from build123d import *

# Parameters (mm, degrees)
SKETCH1_W           = 2.9718
SKETCH1_H           = 12.7
SKETCH1_W_2         = 63.5
SKETCH1_H_2         = 31.75
SKETCH1_W_3         = 25.4
SKETCH1_H_3         = 2.739734253
BOSS_EXTRUDE1_DEPTH = 2.9718
CUT_EXTRUDE1_DEPTH  = 3.9718


with BuildPart() as part:
    # Sketch1 → Boss-Extrude1 (new body)
    with BuildSketch(Plane.XY):
        with Locations((-33.2359, 3.175)):
            Rectangle(SKETCH1_W, SKETCH1_H)
        Rectangle(SKETCH1_W_2, SKETCH1_H_2)
        with Locations((33.2359, 3.175)):
            Rectangle(SKETCH1_W, SKETCH1_H)
        with Locations((0, -17.244867127)):
            Rectangle(SKETCH1_W_3, SKETCH1_H_3)
    extrude(amount=BOSS_EXTRUDE1_DEPTH)

    # Sketch2 → Cut-Extrude1 (cut, through all)
    with BuildSketch(Plane(origin=(0, 0, 0), x_dir=(-1, 0, 0), z_dir=(0, 0, -1))):
        with BuildLine():
            ThreePointArc((34.7218, 2.836359793), (34.750345047, 3.00461162), (34.7599, 3.175))
            ThreePointArc((34.7599, 3.175), (34.750345047, 3.34538838), (34.7218, 3.513640207))
            Line((34.7218, 3.513640207), (34.7218, 2.836359793))
        make_face()
        with BuildLine():
            Line((34.7218, 2.836359793), (34.7218, 3.513640207))
            ThreePointArc((34.7218, 3.513640207), (31.7119, 3.175), (34.7218, 2.836359793))
        make_face()
        with BuildLine():
            ThreePointArc((-34.7218, 2.836359793), (-33.06551162, 1.660554953), (-31.7119, 3.175))
            ThreePointArc((-31.7119, 3.175), (-33.06551162, 4.689445047), (-34.7218, 3.513640207))
            Line((-34.7218, 3.513640207), (-34.7218, 2.836359793))
        make_face()
        with BuildLine():
            Line((-34.7218, 2.836359793), (-34.7218, 3.513640207))
            ThreePointArc((-34.7218, 3.513640207), (-34.7599, 3.175), (-34.7218, 2.836359793))
        make_face()
        Polygon((-31.75, -8.001), (-31.75, -11.049), (-24.5618, -11.049), (-24.5618, -12.7), (-22.0218, -12.7), (-22.0218, -6.35), (-24.5618, -6.35), (-24.5618, -8.001), align=None)
        with BuildLine():
            ThreePointArc((0.667862303, -18.614734253), (1.29236182, -18.052565663), (1.524, -17.244867127))
            ThreePointArc((1.524, -17.244867127), (-0.807698536, -15.952505306), (-0.667862303, -18.614734253))
            Line((-0.667862303, -18.614734253), (0.667862303, -18.614734253))
        make_face()
        with BuildLine():
            Line((0.667862303, -18.614734253), (-0.667862303, -18.614734253))
            ThreePointArc((-0.667862303, -18.614734253), (0, -18.768867127), (0.667862303, -18.614734253))
        make_face()
        Polygon((31.75, -11.049), (24.5618, -11.049), (24.5618, -12.7), (22.0218, -12.7), (22.0218, -6.35), (24.5618, -6.35), (24.5618, -8.001), (31.75, -8.001), align=None)
    extrude(amount=-CUT_EXTRUDE1_DEPTH, mode=Mode.SUBTRACT)


solid = part.part
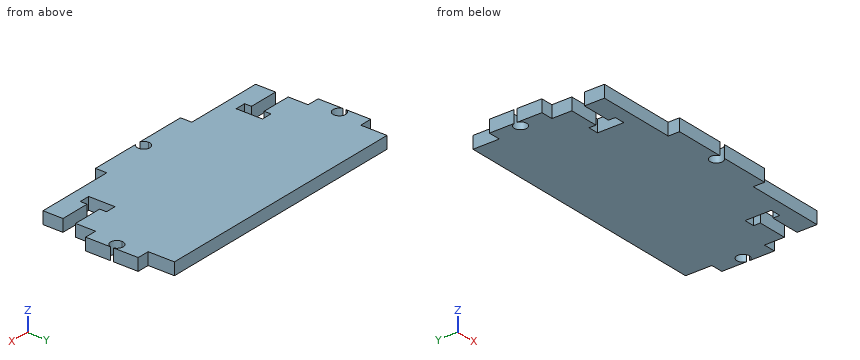
For this review, take the finished solid that the model builds, in its own axes (mm). Coordinates: 2 decimals unless noted, no trailing zeros. Loops run counter-clockwise (first coordinate to the right, second up) from the corner with the lowest first, then second, coordinate; pieces in that order, holes last. Notation, with made-up numbers: (7.5, -23) -> (15.5, -23) arc R13 cw to (15.5, 1) -> close; hole circle Ø1 at (75, 42). An arc over 180 degrees is marked (long way). Write each question's results on one line, items separated by ' | '.
Q1. To check wall thickness, follow line 1 along X through (y, z) = (-11.5, 1.85); line 2 along Y through (x, z) = (-27, 1.2) (3 decimals); line 3 along Y through (x, z) = (21, 1.55) (3 decimals). State the ranges of each line that lie inside material, in increasing order. Write a range as [from, to].
Taken from the geometry:
line 1: [-31.75, -24.56], [-22.02, 22.02], [24.56, 31.75] | line 2: [-15.875, -11.049], [-8.001, 15.875] | line 3: [-15.875, 15.875]
Q2. Add section A-A, the plane x = 26. State the section outline as (y, z) points (3 decimals).
Taken from the geometry:
outline: (-15.875, 0) -> (-11.049, 0) -> (-11.049, 2.972) -> (-15.875, 2.972) -> close; (-8.001, 0) -> (15.875, 0) -> (15.875, 2.972) -> (-8.001, 2.972) -> close
Q3. Add section C-C, the plane y = 11.5. State the section outline as (x, z) points.
Taken from the geometry:
outline: (-31.75, 0) -> (31.75, 0) -> (31.75, 2.97) -> (-31.75, 2.97) -> close
Q4. For pin 1 Ø1.4 at (y, z) = (-17.5, 1.5) entering from -X; pin 2 Ø0.9 at (y, z) = (-10, 1.5) entering from +X; pin 3 Ø0.8 at (y, z) = (-12, 1) entering from +X, all flat-tipped, find the tip position at first contact; note any pin that passes through.
Taken from the geometry:
pin 1: x = -12.7 | pin 2: x = 22.02 | pin 3: x = 31.75
Q5. Add section B-B, the plane x = -13.5. State the section outline as (y, z) points (3 decimals).
Taken from the geometry:
outline: (-15.875, 0) -> (15.875, 0) -> (15.875, 2.972) -> (-15.875, 2.972) -> close
